from build123d import *

# Parameters (mm, degrees)
F0_R     = 2.54
F1_DEPTH = 3.048


with BuildPart() as f1:
    # F0 (on Front) → F1 (new body)
    with BuildSketch(Plane.XZ):
        with BuildLine():
            ThreePointArc((-42.1443581445, 65.6977605384), (-39.2914232505, 59.08092793), (-32.6211089313, 56.3553787816))
            ThreePointArc((-32.6211089313, 56.3553787816), (-25.9507946121, 59.08092793), (-23.0978597181, 65.6977605384))
            Line((-23.0978597181, 65.6977605384), (-23.4511180552, 68.456595452))
            ThreePointArc((-23.4511180552, 68.456595452), (-34.0117887591, 75.3033100992), (-42.1443581445, 65.6977605384))
        make_face()
        with BuildLine():
            ThreePointArc((-29.4461089313, 65.8803787816), (-30.376044901, 63.6353147513), (-32.6211089313, 62.7053787816))
            ThreePointArc((-32.6211089313, 62.7053787816), (-34.8661729616, 68.1254428119), (-29.4461089313, 65.8803787816))
        make_face(mode=Mode.SUBTRACT)
        with BuildLine():
            ThreePointArc((-23.0978597181, 65.6977605384), (-25.9507946121, 59.08092793), (-32.6211089313, 56.3553787816))
            Line((-32.6211089313, 56.3553787816), (-32.6211089313, 30.9553787816))
            ThreePointArc((-32.6211089313, 30.9553787816), (-22.1328460742, 26.997256193), (-16.8746720522, 17.0966502448))
            Line((-16.8746720522, 17.0966502448), (-23.0978597181, 65.6977605384))
        make_face()
        with BuildLine():
            Line((-32.6211089313, 30.9553787816), (-32.6211089313, 56.3553787816))
            ThreePointArc((-32.6211089313, 56.3553787816), (-39.2914232505, 59.08092793), (-42.1443581445, 65.6977605384))
            Line((-42.1443581445, 65.6977605384), (-48.3675458104, 17.0966502448))
            ThreePointArc((-48.3675458104, 17.0966502448), (-43.1093717885, 26.997256193), (-32.6211089313, 30.9553787816))
        make_face()
        with Locations((-37.2888706625, 51.6055787816)):
            Circle(F0_R, mode=Mode.SUBTRACT)
        with BuildLine():
            ThreePointArc((-16.8746720522, 17.0966502448), (-22.1328460742, 26.997256193), (-32.6211089313, 30.9553787816))
            Line((-32.6211089313, 30.9553787816), (-32.6211089313, 18.2553787816))
            ThreePointArc((-32.6211089313, 18.2553787816), (-30.376044901, 17.3254428119), (-29.4461089313, 15.0803787816))
            ThreePointArc((-29.4461089313, 15.0803787816), (-30.376044901, 12.8353147513), (-32.6211089313, 11.9053787816))
            Line((-32.6211089313, 11.9053787816), (-32.6211089313, -0.7946212184))
            ThreePointArc((-32.6211089313, -0.7946212184), (-23.4929168915, 2.0922405361), (-17.6846402517, 9.7028767237))
            Line((-17.6846402517, 9.7028767237), (-16.8746720522, 17.0966502448))
        make_face()
        with BuildLine():
            Line((-32.6211089313, 18.2553787816), (-32.6211089313, 30.9553787816))
            ThreePointArc((-32.6211089313, 30.9553787816), (-43.1093717885, 26.997256193), (-48.3675458104, 17.0966502448))
            Line((-48.3675458104, 17.0966502448), (-47.7009565636, 10.1191470405))
            ThreePointArc((-47.7009565636, 10.1191470405), (-41.9285272391, 2.2200681538), (-32.6211089313, -0.7946212184))
            Line((-32.6211089313, -0.7946212184), (-32.6211089313, 11.9053787816))
            ThreePointArc((-32.6211089313, 11.9053787816), (-35.7961089313, 15.0803787816), (-32.6211089313, 18.2553787816))
        make_face()
        with BuildLine():
            Line((-23.4511180552, 68.456595452), (-23.0978597181, 65.6977605384))
            ThreePointArc((-23.0978597181, 65.6977605384), (-23.0965466381, 65.7890654638), (-23.0961089313, 65.8803787816))
            ThreePointArc((-23.0961089313, 65.8803787816), (-23.1852785997, 67.1806598869), (-23.4511180552, 68.456595452))
        make_face()
        with BuildLine():
            Line((-22.1190817772, -30.7768067438), (-17.6846402517, 9.7028767237))
            ThreePointArc((-17.6846402517, 9.7028767237), (-23.4929168915, 2.0922405361), (-32.6211089313, -0.7946212184))
            Line((-32.6211089313, -0.7946212184), (-32.6211089313, -38.9752205832))
            ThreePointArc((-32.6211089313, -38.9752205832), (-25.9429091979, -41.741421485), (-23.1767082961, -48.4196212184))
            Line((-23.1767082961, -48.4196212184), (3.8913910687, -48.4196212184))
            ThreePointArc((3.8913910687, -48.4196212184), (6.3118425433, -42.7129512772), (12.0970179835, -40.4866511436))
            Line((12.0970179835, -40.4866511436), (-14.4847162499, -39.5882135694))
            ThreePointArc((-14.4847162499, -39.5882135694), (-20.2247777383, -36.848527779), (-22.1190817772, -30.7768067438))
        make_face()
        with BuildLine():
            ThreePointArc((-32.6211089313, -0.7946212184), (-41.9285272391, 2.2200681538), (-47.7009565636, 10.1191470405))
            Line((-47.7009565636, 10.1191470405), (-42.0227039741, -49.3177938133))
            ThreePointArc((-42.0227039741, -49.3177938133), (-39.609649737, -42.0669052034), (-32.6211089313, -38.9752205832))
            Line((-32.6211089313, -38.9752205832), (-32.6211089313, -0.7946212184))
        make_face()
        with BuildLine():
            ThreePointArc((-32.6211089313, -38.9752205832), (-39.609649737, -42.0669052034), (-42.0227039741, -49.3177938133))
            ThreePointArc((-42.0227039741, -49.3177938133), (-38.9622943166, -55.4186262383), (-32.5899670381, -57.86397051))
            Line((-32.5899670381, -57.86397051), (-32.0140661705, -57.8444927))
            ThreePointArc((-32.0140661705, -57.8444927), (-25.7316293285, -54.8796346984), (-23.1767082961, -48.4196212184))
            ThreePointArc((-23.1767082961, -48.4196212184), (-25.9429091979, -41.741421485), (-32.6211089313, -38.9752205832))
        make_face()
        with BuildLine():
            ThreePointArc((-32.6211089313, -45.2446212184), (-30.376044901, -46.1745571881), (-29.4461089313, -48.4196212184))
            ThreePointArc((-29.4461089313, -48.4196212184), (-34.8661729616, -50.6646852487), (-32.6211089313, -45.2446212184))
        make_face(mode=Mode.SUBTRACT)
        with BuildLine():
            Line((-32.0140661705, -57.8444927), (-32.5899670381, -57.86397051))
            ThreePointArc((-32.5899670381, -57.86397051), (-32.30186802, -57.8586247993), (-32.0140661705, -57.8444927))
        make_face()
        with BuildLine():
            Line((3.8913910687, -48.4196212184), (-23.1767082961, -48.4196212184))
            ThreePointArc((-23.1767082961, -48.4196212184), (-25.7316293285, -54.8796346984), (-32.0140661705, -57.8444927))
            Line((-32.0140661705, -57.8444927), (12.0971955203, -56.3525852906))
            ThreePointArc((12.0971955203, -56.3525852906), (6.3119064002, -54.126352894), (3.8913910687, -48.4196212184))
        make_face()
        with BuildLine():
            ThreePointArc((19.7663910687, -48.4196212184), (17.5355610099, -42.902572693), (12.0970179835, -40.4866511436))
            ThreePointArc((12.0970179835, -40.4866511436), (6.3118425433, -42.7129512772), (3.8913910687, -48.4196212184))
            ThreePointArc((3.8913910687, -48.4196212184), (6.3119064002, -54.126352894), (12.0971955203, -56.3525852906))
            ThreePointArc((12.0971955203, -56.3525852906), (17.5356227443, -53.9366058869), (19.7663910687, -48.4196212184))
        make_face()
        with BuildLine():
            ThreePointArc((15.0038910687, -48.4196212184), (11.8288910687, -51.5946212184), (8.6538910687, -48.4196212184))
            ThreePointArc((8.6538910687, -48.4196212184), (11.8288910687, -45.2446212184), (15.0038910687, -48.4196212184))
        make_face(mode=Mode.SUBTRACT)
    extrude(amount=F1_DEPTH)


solid = f1.part
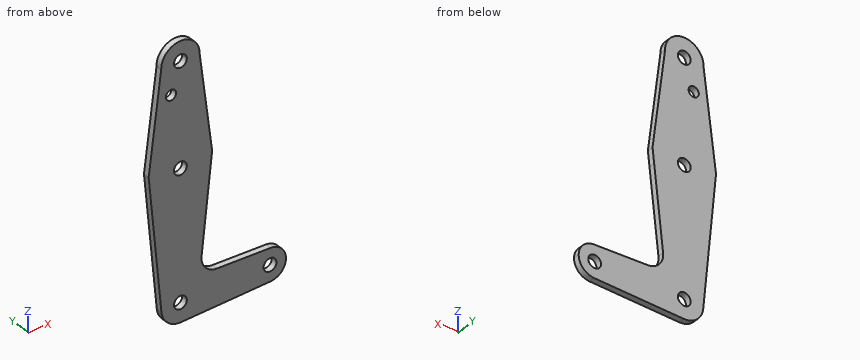
Could you check a few things on this model? Use its own coordinates, in mm. Give positions to 0.01 mm unless a question says otherwise; leave off trailing zeros. Order: outer loops, then holes, each group sorted by start corner. A loop starts at its lowest first (then second) coordinate and runs counter-clockwise, first axis right, second up.
1. Suppose I cut it at B-B (z = -6.5). List the corners of the cut face in (x, y) for me.
2. Suppose I cut it at A-A (y = -1.85). Give the number of separate pieces and of enclosed holes in the cut face, plus the area to 3 significant figures.
3. Will this pin go through, and if not, where does the flat tip stop? P1, Ø1, axis at x = 5, y = -2.5, coming from the -Z side.
4. Suppose I cut it at C-C (x = -25). List the corners of the cut face in (y, z) for me, plus the area to 3 significant figures.
5. I need wall thicknesses on L1, parallel to X at y = -0.45, z = 53.5; L2, parallel to X at y = -0.75, z = 23.5; L3, parallel to Z at x = -12, y = -1.05. Which ranges of each line are inside material? Lowest first, please.
Solved:
1. outline: (-46.11, -3.05) - (-19.46, -3.05) - (-19.46, 0) - (-46.11, 0) - close
2. separate pieces: 1
2. enclosed holes: 5
2. area: 3,720 mm2
3. P1: stops at z = -56.61
4. outline: (-3.05, -57.61) - (0, -57.61) - (0, 71.59) - (-3.05, 71.59) - close
4. area: 394 mm2
5. L1: x = -43.71 to -38.98, -35.6 to -21.54
5. L2: x = -47.55 to -17.69
5. L3: z = -57.17 to -39.67
